The drawing under review shows one solid part. Ordinate dimensions are in mm from its lowest x, y, z. A direction names the side the tool comes from. Coordinates: 2 decimals unless noted, no trailing zeros. Order: outer loops, then holes, each group sorted by start corner. A loop starts at its lowest first (then second) coordinate and runs counter-clockwise, first axis right, second up. Notation, with made-up numbers: (58, 63.5) -> (76, 63.5) arc R15 ccw to (76, 91.5) -> close; hole circle Ø4 at (-17.5, 46). An arc over 180 degrees is marked (long way). Put each result on its own line as item: value.
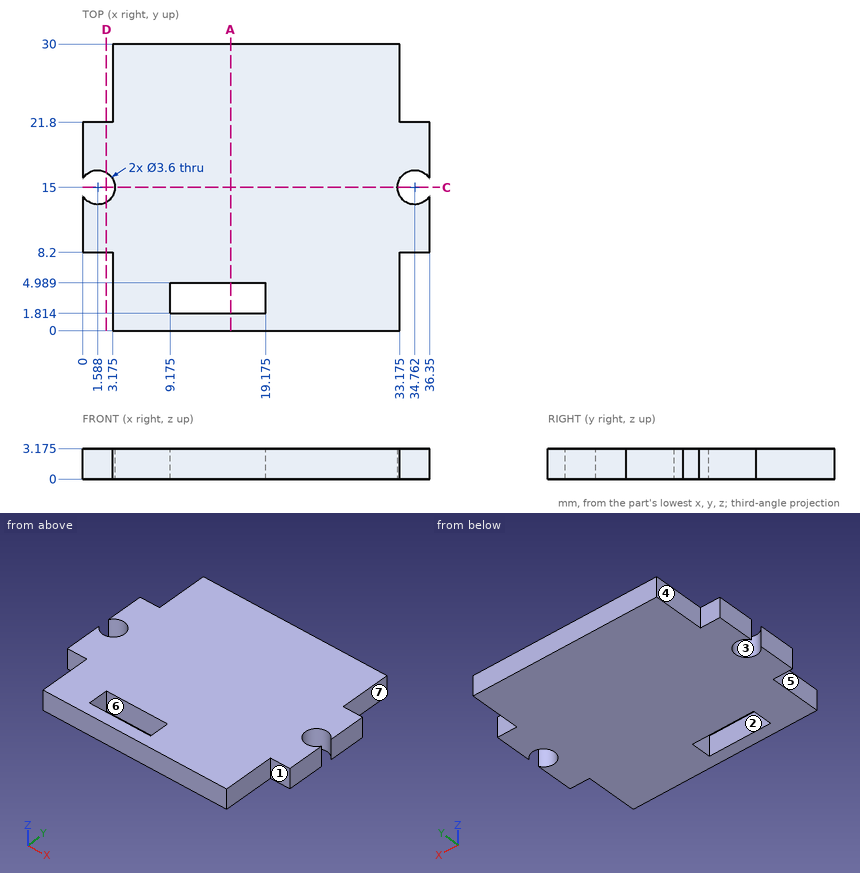
Item 1: Consider section D-D on x = 2.5. Write out the cut boundary in (y, z) (1 decimal).
Answers below:
outline: (8.2, 0) -> (13.4, 0) -> (13.4, 3.2) -> (8.2, 3.2) -> close; (16.6, 0) -> (21.8, 0) -> (21.8, 3.2) -> (16.6, 3.2) -> close
Item 2: Mouldability with a two-part tool opening along Y and no side actions: class the marked faces 1, 2, 3 and 4 as +Y half, -Y half, draft (parallel to the pull), parting line (faces both ways), or undercut.
Answers below:
face 1: -Y half
face 2: undercut
face 3: undercut
face 4: draft
Item 3: Consider section C-C on y = 15. Write out the cut boundary in (x, z) (1 decimal).
Answers below:
outline: (3.4, 0) -> (33, 0) -> (33, 3.2) -> (3.4, 3.2) -> close
Item 4: For line 1 (X direction, y = 4, z = 0.2) (1 decimal); line 2 (Y direction, x = 11, z = 0.9) (1 decimal); line 3 (X direction, y = 15, z = 1.5), list the stretches that pass through material, from the lowest coordinate up. Write a range as from..to.
Answers below:
line 1: 3.2..9.2, 19.2..33.2
line 2: 0..1.8, 5..30
line 3: 3.39..32.96
Item 5: For pin 1 Ø1 at (x, z) = (34, 1) entering from -Y; pin 2 Ø1 at (y, z) = (4, 1) entering from -X (1 decimal); pin 3 Ø1.6 at (y, z) = (2.5, 1) entering from +X (1 decimal), all flat-tipped, find the tip position at first contact; note any pin that passes through.
Answers below:
pin 1: y = 8.2
pin 2: x = 3.2
pin 3: x = 33.2
Item 6: Consider section A-A on x = 15.5. Write out the cut boundary in (y, z) (1 decimal).
Answers below:
outline: (0, 0) -> (1.8, 0) -> (1.8, 3.2) -> (0, 3.2) -> close; (5, 0) -> (30, 0) -> (30, 3.2) -> (5, 3.2) -> close
Item 7: For the marked faces 5, 6 and 7, list the 3-axis set-ups (+Z, -Z, +X, -X, +Y, -Y) from which the entire face can be reached by the end or side of a thin tool; tool diameter is ignored.
Answers below:
face 5: +Z, -Z, -X, -Y
face 6: +Z, -Z
face 7: +Z, -Z, +X, +Y
